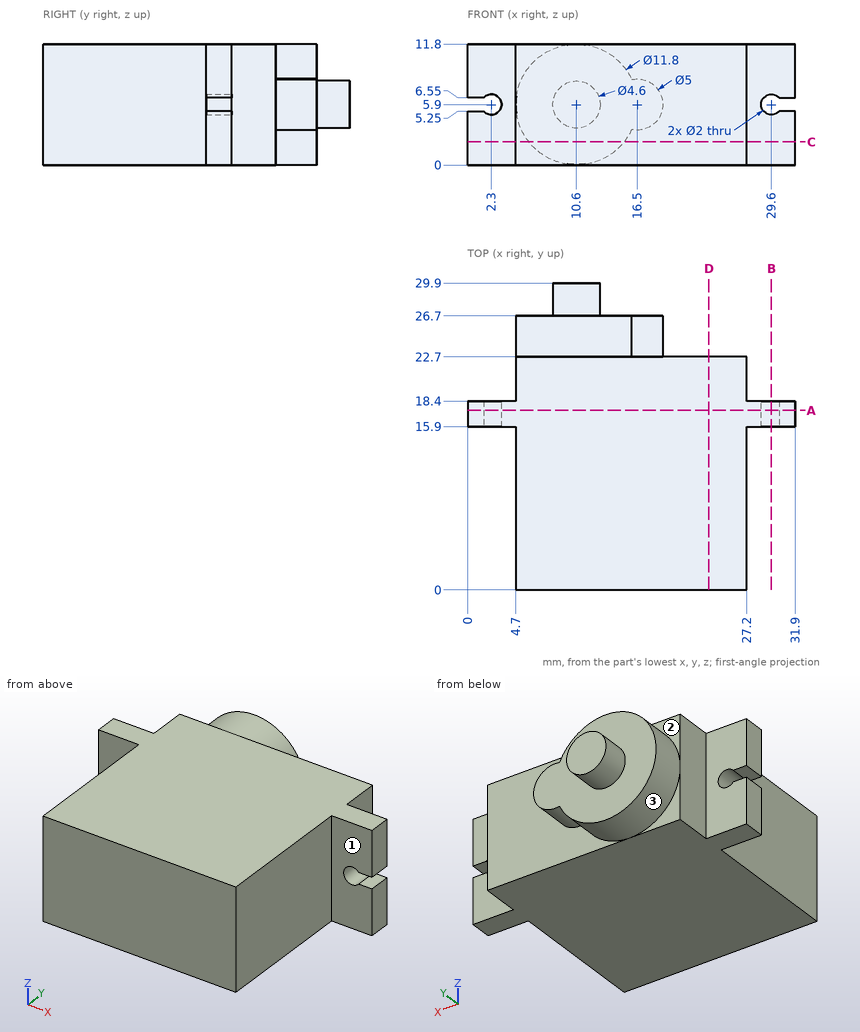
Here's the drawing with two shaded views (mm, measured from the low corner). I have some questions. A direction names the side the tool comes from. Round coordinates to 2 decimals unless told otherwise and drop trailing zeros. Loops run counter-clockwise (first coordinate to the right, second up) from the corner with the lowest first, then second, coordinate; pieces in that order, holes last.
Item 1: Will these pins go through, and if not, where does the flat tip stop? pin 1 Ø1.2 at (x, z) = (29.6, 5.9) entering from -Y; pin 2 Ø2.5 at (x, z) = (2.3, 5.9) entering from -Y; pin 3 Ø6 at (y, z) = (11, 6) entering from +X; pin 4 Ø6 at (y, z) = (22.5, 2.5) entering from -X.
Item 2: Please list where these lines run through material, in increasing order: L1, parallel to Z at x = 2.3, y = 16.95; L2, parallel to X at y = 3.25, z = 9.5; L3, parallel to X at y = 16.5, z = 5.9.
Item 3: Suppose I cut it at D-D, the plane x = 23.5. Write out the boundary of the cut face in (y, z).
Item 4: Suppose I cut it at B-B, the plane x = 29.6. Write out the boundary of the cut face in (y, z).
Item 5: Suppose I cut it at A-A, the plane y = 17.5. Write out the boundary of the cut face in (x, z).
Item 6: Which directions (+Z, -Z, +X, -X, +Y, -Y) give clear straight access to the entire face, cutting with the end or side of a thin tool? Please do the marked faces 1, 2 and 3.
Item 7: Suppose I cut it at C-C, the plane z = 2.25. Write out the boundary of the cut face in (x, y).
Reported:
1. pin 1: passes through
1. pin 2: stops at y = 15.9
1. pin 3: stops at x = 27.2
1. pin 4: stops at x = 4.7
2. L1: z = 0 to 4.9, 6.9 to 11.8
2. L2: x = 4.7 to 27.2
2. L3: x = 3.3 to 28.6
3. outline: (0, 0) - (22.7, 0) - (22.7, 11.8) - (0, 11.8) - close
4. outline: (15.9, 0) - (18.4, 0) - (18.4, 4.9) - (15.9, 4.9) - close; (15.9, 6.9) - (18.4, 6.9) - (18.4, 11.8) - (15.9, 11.8) - close
5. outline: (0, 0) - (31.9, 0) - (31.9, 5.25) - (30.36, 5.25) arc R1 cw (long way) to (30.36, 6.55) - (31.9, 6.55) - (31.9, 11.8) - (0, 11.8) - (0, 6.55) - (1.54, 6.55) arc R1 cw (long way) to (1.54, 5.25) - (0, 5.25) - close
6. face 1: +Z, -Z, +X, -Y
6. face 2: +Z, -X, +Y
6. face 3: +Y
7. outline: (0, 15.9) - (4.7, 15.9) - (4.7, 0) - (27.2, 0) - (27.2, 15.9) - (31.9, 15.9) - (31.9, 18.4) - (27.2, 18.4) - (27.2, 22.7) - (15.24, 22.7) - (15.24, 26.7) - (5.96, 26.7) - (5.96, 22.7) - (4.7, 22.7) - (4.7, 18.4) - (0, 18.4) - close
